Design review of the part built by this model. Coordinates are the model's own, in mm. A direction names the side the tool comes from. Give positions to 0.01 mm unless a question says otherwise; leave off trailing zeros. Loops run counter-clockwise (first coordinate to the right, second up) from the corner with the lowest first, then second, coordinate; pieces in that order, holes last.
from build123d import *

# Parameters (mm, degrees)
F1_DEPTH  = 6
F2_W      = 18
F2_H      = 36
F3_DEPTH  = 8
F4_SIZE2  = 7.99999
F4_SIZE   = 4.99999
F6_DEPTH  = 1
F7_R      = 8.4004464167
F8_DEPTH  = 2
F9_R      = 4
F10_DEPTH = 25
F11_R     = 5


# Not quite as in the source:
# - a fillet or chamfer is up to 0.001 mm smaller than in the source, because OpenCascade refuses the exact size


with BuildPart() as f1:
    # F0 (on Top) → F1 (new body)
    with BuildSketch(Plane.XY):
        Polygon((7.5, 100), (-7.5, 100), (-20.6415709108, 31.671449542), (-11.5, 13), (-11.5, -13), (-20.6415709108, -31.671449542), (-7.5, -100), (7.5, -100), (20.6415709108, -31.671449542), (11.5, -13), (11.5, 13), (20.6415709108, 31.671449542), align=None)
        with BuildLine():
            ThreePointArc((0, -88), (-1.767766953, -87.267766953), (-2.5, -85.5))
            Line((-2.5, -85.5), (-2.5, -27.5))
            ThreePointArc((-2.5, -27.5), (-1.767766953, -25.732233047), (0, -25))
            ThreePointArc((0, -25), (1.767766953, -25.732233047), (2.5, -27.5))
            Line((2.5, -27.5), (2.5, -85.5))
            ThreePointArc((2.5, -85.5), (1.767766953, -87.267766953), (0, -88))
        make_face(mode=Mode.SUBTRACT)
        Polygon((-6.5, 3.7527767497), (0, 7.5055534995), (6.5, 3.7527767497), (6.5, -3.7527767497), (0, -7.5055534995), (-6.5, -3.7527767497), align=None, mode=Mode.SUBTRACT)
        with BuildLine():
            ThreePointArc((0, 25), (-1.767766953, 25.732233047), (-2.5, 27.5))
            Line((-2.5, 27.5), (-2.5, 85.5))
            ThreePointArc((-2.5, 85.5), (-1.767766953, 87.267766953), (0, 88))
            ThreePointArc((0, 88), (1.767766953, 87.267766953), (2.5, 85.5))
            Line((2.5, 85.5), (2.5, 27.5))
            ThreePointArc((2.5, 27.5), (1.767766953, 25.732233047), (0, 25))
        make_face(mode=Mode.SUBTRACT)
    extrude(amount=F1_DEPTH)

    # F2 (on face) → F3 (join)
    with BuildSketch(Plane.XY.offset(6)):
        Rectangle(F2_W, F2_H)
    extrude(amount=F3_DEPTH)

    # F4 (size 5 and 8 in the source; OpenCascade refuses exactly that, so slightly less here)
    f4_edges = [f1.edges().sort_by_distance(p)[0] for p in [
        (0, -18, 14),
        (0, 18, 14),
    ]]
    f4_side = f1.faces().sort_by_distance((0, 0, 14))[0]
    chamfer(f4_edges, length=F4_SIZE, length2=F4_SIZE2, reference=f4_side)

    # F5 (on face) → F6 (cut)
    with BuildSketch(Plane(origin=(0, 0, 6), x_dir=(1, 0, 0), z_dir=(0, 0, -1))):
        Polygon((6.5, 3.7527767497), (0, 7.5055534995), (-6.5, 3.7527767497), (-6.5, -3.7527767497), (0, -7.5055534995), (6.5, -3.7527767497), align=None)
    extrude(amount=-F6_DEPTH, mode=Mode.SUBTRACT)

    # F7 (on face) → F8 (cut)
    with BuildSketch(Plane.XY.offset(14)):
        Circle(F7_R)
    extrude(amount=-F8_DEPTH, mode=Mode.SUBTRACT)

    # F9 (on face) → F10 (cut)
    with BuildSketch(Plane.XY.offset(12)):
        Circle(F9_R)
    extrude(amount=-F10_DEPTH, mode=Mode.SUBTRACT)

    # F11
    f11_edges = [f1.edges().sort_by_distance(p)[0] for p in [
        (0, -100, 6),
        (0, 100, 6),
    ]]
    fillet(f11_edges, radius=F11_R)


solid = f1.part
Q1. Draft analysis for pull direction Y (two halves, no side actions). For faces 6 (the face through (-13.98, 66.31, 2.96)), 7 (the face through (-3.3, 5.6, 3.5)), 8 (the face through (-0.126, -15.535, 9.944)), state which applies: pulls with the +Y half, pulls with the -Y half, needs draft (parallel to the pull), parting line crosses it, or undercut.
Results:
face 6: pulls with the +Y half
face 7: undercut
face 8: pulls with the -Y half
Q2. Wall thickness on line 1 (Z direction, x = -3, y = -67); line 2 (X direction, y = 54, z = 2.5); line 3 (X direction, y = 41, z = 4.25): over which ranges is each line inside the solid? List them lowest first.
Results:
line 1: z = 0 to 6
line 2: x = -16.35 to -2.5, 2.5 to 16.35
line 3: x = -18.85 to -2.5, 2.5 to 18.85
Q3. Take a section at B-B (z = 4.25). Give the boundary of the cut face in (x, y), plus the area to 3 significant figures.
Results:
outline: (-20.64, -31.67) - (-7.73, -98.8) - (7.73, -98.8) - (20.64, -31.67) - (11.5, -13) - (11.5, 13) - (20.64, 31.67) - (7.73, 98.8) - (-7.73, 98.8) - (-20.64, 31.67) - (-11.5, 13) - (-11.5, -13) - close; hole (-6.5, -3.75) - (0, -7.51) - (6.5, -3.75) - (6.5, 3.75) - (0, 7.51) - (-6.5, 3.75) - close; hole (-2.5, -85.5) arc R2.5 ccw to (2.5, -85.5) - (2.5, -27.5) arc R2.5 ccw to (-2.5, -27.5) - close; hole (-2.5, 27.5) arc R2.5 ccw to (2.5, 27.5) - (2.5, 85.5) arc R2.5 ccw to (-2.5, 85.5) - close
area: 4,840 mm2
Q4. Take a section at A-A (y = 0). Give the boundary of the cut face in (x, z), plus the area to 3 significant figures.
Results:
outline: (-11.5, 0) - (-6.5, 0) - (-6.5, 7) - (-4, 7) - (-4, 12) - (-8.4, 12) - (-8.4, 14) - (-9, 14) - (-9, 6) - (-11.5, 6) - close; (4, 7) - (6.5, 7) - (6.5, 0) - (11.5, 0) - (11.5, 6) - (9, 6) - (9, 14) - (8.4, 14) - (8.4, 12) - (4, 12) - close
area: 117 mm2
Q5. Insertion check: pin 1 (3.5 mm diameter, centred on y = 1.5, z = 4.5, fed in from -X); pin 2 (6 mm diameter, centred on x = -14, y = -66, fed in from +Z); pin 3 (2 mm diameter, centred on y = -61.5, z = 4.5, fed in from +X); pin 4 (10 mm diameter, centred on x = -1.5, y = -18, fed in from -Z). Each pin has a flat end and moves straight along its axis. Give the tip position at first contact, or say it passes through.
Results:
pin 1: stops at x = -11.5
pin 2: stops at z = 6
pin 3: stops at x = 15.1
pin 4: stops at z = 0
Q6. Take a section at C-C (y = -41). Give the boundary of the cut face in (x, z).
Results:
outline: (-18.85, 0) - (-2.5, 0) - (-2.5, 6) - (-18.85, 6) - close; (2.5, 0) - (18.85, 0) - (18.85, 6) - (2.5, 6) - close
Q7. Tool access review of faces 1 (the face through (-16.01, -22.21, 2.96)), 2 (the face through (-6.67, -5.11, 13.01)), 3 (the face through (9, 0, 10)), 4 (the face through (-9, 0, 10)), 5 (the face through (3.3, -5.6, 3.5)): name each direction out of +Z, -Z, +X, -X, +Y, -Y from which nothing blocks a thin tool from reaching the whole face with its end or side.
Results:
face 1: +Z, -Z, -X
face 2: +Z
face 3: +Z, +X, +Y, -Y
face 4: +Z, -X, +Y, -Y
face 5: -Z
